Job drawing, mm, ordinate dimensions from the low corner. One solid piece. Coordinates: 2 decimals unless noted, no trailing zeros. Order: outer loops, then holes, each group sorted by start corner. A loop starts at its lowest first (then second) coordinate and runs counter-clockwise, first axis right, second up. Notation, with made-up numbers: (58.5, -39.75) - (68.5, -39.75) arc R21 ccw to (68.5, -18.75) - close; hole circle Ø9 at (46, -21). An arc over 180 degrees is marked (long way). Return JSON: item names as keys, results as strings.
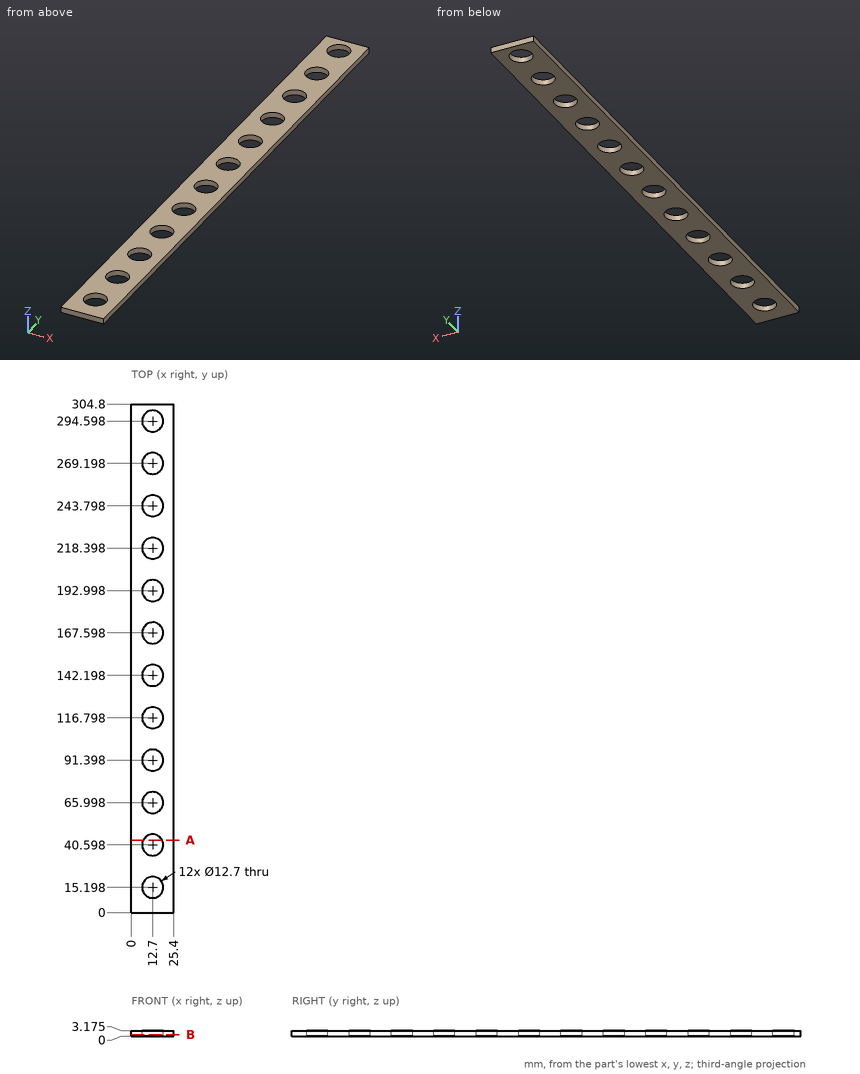
1. Drop a flat-ended pin along its axis: pin 1 (7.5 mm diameter, centred on x = 12.7, y = 40.6, fed in from -Z). Give the stop position or say it passes through.
Check values:
{"pin 1": "through"}
2. Cut at A-A on y = 43.5. Give the cut face in (x, z) (1 decimal), plus the area to 3 significant figures.
Check values:
{"outline": "(0, 0) - (7.1, 0) - (7.1, 3.2) - (0, 3.2) - close; (18.3, 0) - (25.4, 0) - (25.4, 3.2) - (18.3, 3.2) - close", "area": "44.8 mm²"}
3. Cut at B-B on z = 0.8. State how many separate pieces and enclosed holes the cut face has, plus the area to 3 significant figures.
Check values:
{"separate pieces": "1", "enclosed holes": "12", "area": "6,220 mm²"}
4. Probe L1, parallel to X at y = 143, z = 0.7; L2, parallel to X at y = 217, z = 0.7 (1 decimal). List the from-to ranges inside material, lowest first.
Check values:
{"L1": "0 to 6.4, 19 to 25.4", "L2": "0 to 6.5, 18.9 to 25.4"}
